from build123d import *

# Parameters (mm, degrees)
ESBO_O1_R                = 3.15
ESBO_O1_R_2              = 1.6
RESSALTO_EXTRUS_O1_DEPTH = 6
FILETE2_R                = 8
FILETE3_R                = 4
FILETE4_R                = 20


with BuildPart() as part:
    # Esboço1 → Ressalto-extrusão1 (new body)
    with BuildSketch(Plane.XY):
        Polygon((22, 0), (9, 0), (9, -19), (0, -19), (0, -29), (6, -29), (6, -39), (0, -39), (0, -45), (32.15, -45), (32.15, -15), (45, -15), (45, 0), (32, 0), (32, 6), (22, 6), align=None)
        with Locations((22.15, -27.680849585)):
            Circle(ESBO_O1_R, mode=Mode.SUBTRACT)
        with Locations((19, -8)):
            Circle(ESBO_O1_R_2, mode=Mode.SUBTRACT)
        with Locations((39, -8)):
            Circle(ESBO_O1_R_2, mode=Mode.SUBTRACT)
    extrude(amount=RESSALTO_EXTRUS_O1_DEPTH)

    # Filete2
    filete2_edges = [part.edges().sort_by_distance(p)[0] for p in [
        (45, -15, 3),
    ]]
    fillet(filete2_edges, radius=FILETE2_R)

    # Filete3
    filete3_edges = [part.edges().sort_by_distance(p)[0] for p in [
        (32.15, -15, 3),
    ]]
    fillet(filete3_edges, radius=FILETE3_R)

    # Filete4
    filete4_edges = [part.edges().sort_by_distance(p)[0] for p in [
        (32.15, -45, 3),
    ]]
    fillet(filete4_edges, radius=FILETE4_R)


solid = part.part
Could you check a few things on this model? Use its own coordinates, in mm. A direction names the side the tool comes from. Coordinates: 2 decimals unless noted, no trailing zeros. Order: outer loops, then holes, each group sorted by start corner. A loop starts at its lowest first (then second) coordinate and runs counter-clockwise, first axis right, second up. Notation, with made-up numbers: (33.25, -9.5) -> (63.25, -9.5) arc R18 cw to (63.25, -0.5) -> close; hole circle Ø4 at (46, 64.5). An arc over 180 degrees is marked (long way). One line per item, written item: value. Start each with the question number.
1) I'm going to push flat-ended pins straight in: pin 1 (7 mm diameter, centred on x = 22.15, y = -27.68, fed in from -Z); pin 2 (1 mm diameter, centred on x = 35.5, z = 5, fed in from -Y); pin 3 (0.7 mm diameter, centred on x = 36.5, z = 4.5, fed in from -Y); pin 4 (3 mm diameter, centred on y = -21.5, z = 3, fed in from +X). Where does each tip first touch, or does it pass through?
2) Which directions (+Z, -Z, +X, -X, +Y, -Y) give clear straight access to the entire face, cutting with the end or side of a thin tool? Please do faces 4 (the flat face through (22, -19, 6)), 5 (the flat face through (32.15, -22, 3)), 6 (the flat face through (6, -34, 3)), 7 (the flat face through (22, 3, 3)), 8 (the flat face through (45, -4, 3)).
3) Imagine slicing it at C-C on z = 1.7. List the corners of the cut face in (x, y) for me, plus the area to 3 significant figures.
4) If I drill on L1, parallel to X at y = 3, z = 3.65; L2, parallel to Y at x = 22.15, z = 2; L3, parallel to X at y = -3, z = 0.95, over which ranges is the centre line in solid material (lowest first)? Write a range as [from, to].
5) Imagine slicing it at A-A on y = -9. List the corners of the cut face in (x, z) for me.
6) We'd pull the mould along Y, two halves only. Please class faces 1 (the cylindrical face through (26.447, -38.986, 3.042)), 2 (the flat face through (3, -29, 3)), 3 (the flat face through (27, 6, 3)): +Y half, -Y half, draft (parallel to the pull), parting line (faces both ways), or undercut.
7) Imagine slicing it at B-B on x = 38. List the corners of the cut face in (y, z) for me, plus the area to 3 significant figures.
8) Imagine slicing it at D-D on x = 31. List the corners of the cut face in (y, z) for me.
Answer list:
1. pin 1: stops at z = 0
1. pin 2: stops at y = -15.17
1. pin 3: stops at y = -15
1. pin 4: stops at x = 32.15
2. face 4: +Z, +X, -X, +Y, -Y
2. face 5: +Z, -Z, +X, -Y
2. face 6: +Z, -Z, -X
2. face 7: +Z, -Z, -X, +Y
2. face 8: +Z, -Z, +X, +Y, -Y
3. outline: (0, -45) -> (12.15, -45) arc R20 ccw to (32.15, -25) -> (32.15, -19) arc R4 cw to (36.15, -15) -> (37, -15) arc R8 ccw to (45, -7) -> (45, 0) -> (32, 0) -> (32, 6) -> (22, 6) -> (22, 0) -> (9, 0) -> (9, -19) -> (0, -19) -> (0, -29) -> (6, -29) -> (6, -39) -> (0, -39) -> close; hole circle Ø3.2 at (19, -8); hole circle Ø6.3 at (22.15, -27.68); hole circle Ø3.2 at (39, -8)
3. area: 1,330 mm2
4. L1: x = [22, 32]
4. L2: y = [-42.32, -30.83], [-24.53, 6]
4. L3: x = [9, 45]
5. outline: (9, 0) -> (17.75, 0) -> (17.75, 6) -> (9, 6) -> close; (20.25, 0) -> (37.75, 0) -> (37.75, 6) -> (20.25, 6) -> close; (40.25, 0) -> (44.75, 0) -> (44.75, 6) -> (40.25, 6) -> close
6. face 1: -Y half
6. face 2: undercut
6. face 3: +Y half
7. outline: (-14.94, 0) -> (-9.25, 0) -> (-9.25, 6) -> (-14.94, 6) -> close; (-6.75, 0) -> (0, 0) -> (0, 6) -> (-6.75, 6) -> close
7. area: 74.6 mm2
8. outline: (-31.68, 0) -> (6, 0) -> (6, 6) -> (-31.68, 6) -> close
